from build123d import *

# Parameters (mm, degrees)
F0_W     = 107.95
F0_H     = 31.75
F1_DEPTH = 31.75
F3_DEPTH = 31.751
F5_DEPTH = 31.7506558501


with BuildPart() as f1:
    # F0 (on Front) → F1 (new body)
    with BuildSketch(Plane.XZ):
        with Locations((1.144817099, -4.4740095741)):
            Rectangle(F0_W, F0_H)
    extrude(amount=F1_DEPTH)

    # F2 (on face) → F3 (cut, through all)
    with BuildSketch(Plane.XZ.offset(31.75)):
        with BuildLine():
            ThreePointArc((-34.6886992289, -10.405750614), (-31.724758859, -8.0747267722), (-30.605182901, -4.4740095741))
            ThreePointArc((-30.605182901, -4.4740095741), (-31.724758859, -0.8732923759), (-34.6886992289, 1.4577314658))
            ThreePointArc((-34.6886992289, 1.4577314658), (-43.305182901, -4.4740095741), (-34.6886992289, -10.405750614))
        make_face()
        with BuildLine():
            ThreePointArc((-36.955182901, -19.9203009288), (-52.4014742558, -4.4740095741), (-36.955182901, 10.9722817806))
            Line((-36.955182901, 10.9722817806), (55.119817099, 11.4009904259))
            Line((55.119817099, 11.4009904259), (-52.830182901, 11.4009904259))
            Line((-52.830182901, 11.4009904259), (-52.830182901, -20.3490095741))
            Line((-52.830182901, -20.3490095741), (13.844817099, -20.3490095741))
            Line((13.844817099, -20.3490095741), (13.844817099, -20.1568298366))
            Line((13.844817099, -20.1568298366), (-36.955182901, -19.9203009288))
        make_face()
        Polygon((55.119817099, -10.823906328), (55.119817099, 1.8758871798), (13.844817099, 1.6837074423), (13.844817099, -10.6317265905), align=None)
    extrude(amount=-F3_DEPTH, mode=Mode.SUBTRACT)

    # F4 (on face) → F5 (cut, through all)
    with BuildSketch(Plane(origin=(-0.051887861, 0, 11.1441065064), x_dir=(0.9999891606, 0, 0.0046560304), z_dir=(-0.0046560304, 0, 0.9999891606))):
        with BuildLine():
            ThreePointArc((38.2637782771, -22.1403273388), (43.4058074687, -20.7167652744), (45.6473029929, -15.875))
            ThreePointArc((45.6473029929, -15.875), (35.1887985171, -11.0332347256), (38.2637782771, -22.1403273388))
        make_face()
    extrude(amount=-F5_DEPTH, mode=Mode.SUBTRACT)


solid = f1.part
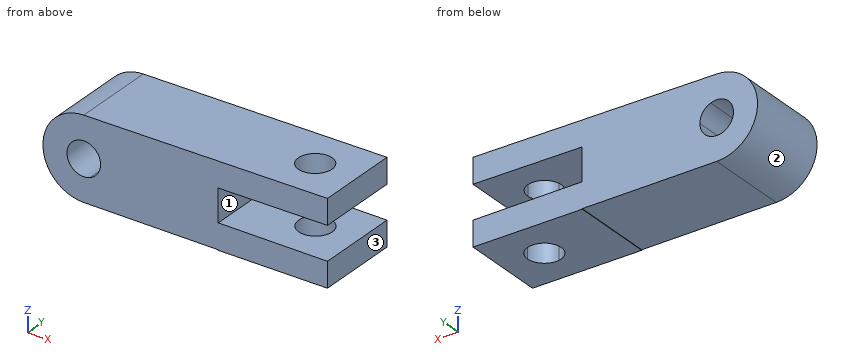
Read the model definition and answer for the solid it produces. Units are mm, in the model's axes. Face numbers are marked on the shaded views. Coordinates: 2 decimals unless noted, no trailing zeros. Write each loop counter-clockwise with the first axis right and the second up, starting at its lowest first coordinate (ties: lowest second). Pieces come first, ordered by that corner, then holes. Notation, with made-up numbers: M 9.25,28.25 L 53.25,28.25 A25 cw 53.25,48.25 Z; hole C -4.75,52 d9. An arc over 180 degrees is marked long. Use a Markdown table: item, result.
Q1. Each of these flat-tipped pins is pushed along its axis until it touches: pin 1 Ø1.5 at (y, z) = (-5.5, -4) entering from +X; pin 2 Ø1 at (x, y) = (-25.5, -6) entering from +Z; pin 3 Ø8 at (x, y) = (14.5, -10.5) entering from +Z; pin 4 Ø5 at (x, z) = (-37, -6.5) entering from +Y. Where does it stop, or does it pass through?
Answer block:
| item | result |
|---|---|
| pin 1 | stops at x = 13.84 |
| pin 2 | stops at z = 11.03 |
| pin 3 | stops at z = 11.23 |
| pin 4 | passes through |
Q2. The part is cut by section D-D, the plane z = -8. Write down the section's boundary in (x, y).
Answer block:
| item | result |
|---|---|
| outline | M -51.99,-31.75 L -42.24,-31.75 L -42.24,0 L -51.99,0 Z; M -31.67,-31.75 L 13.84,-31.75 L 13.84,0 L -31.67,0 Z |
Q3. Determine the mould class of the marked faces 1, 2 and 3 for opening direction Z: released by +Z, released by -Z, zero draft, split by the parting line, or undercut.
Answer block:
| item | result |
|---|---|
| face 1 | undercut |
| face 2 | split by the parting line |
| face 3 | zero draft |
Q4. The part is cut by section C-C, the plane x = -36. Write down the section's boundary in (y, z).
Answer block:
| item | result |
|---|---|
| outline | M -31.75,-19.92 L 0,-19.92 L 0,-10.75 L -31.75,-10.75 Z; M -31.75,1.8 L 0,1.8 L 0,10.98 L -31.75,10.98 Z |
Q5. Straight lines are drawn through the part: L1, parallel to Y at x = 39, z = 5; L2, parallel to Z at x = 50.5, y = -1.5; L3, parallel to Z at x = 41, y = -9. For each, find the intervals that lie inside material, in ascending order. Write a range as [from, to].
Answer block:
| item | result |
|---|---|
| L1 | y = [-31.75, -22.22], [-9.53, 0] |
| L2 | z = [-20.35, -10.8], [1.85, 11.38] |
| L3 | z = [-20.35, -10.76], [1.81, 11.34] |
